The model under review builds one solid part; all positions refer to its coordinate system, in mm. A direction names the side the tool comes from. Coordinates: 2 decimals unless noted, no trailing zeros. Write each loop counter-clockwise with the first axis right and the second up, starting at its lowest first coordinate (ties: lowest second). Pieces come first, ordered by that corner, then holes.
1) Add section B-B, the plane y = -12.5. Give the number of separate pieces and of enclosed holes in the cut face, then the cut area to 3 significant figures.
2) For P1, Ø3, axis at y = -5, z = -3.5, coming from the -X side; P2, Ø4, axis at y = -12.5, z = -2, coming from the +X side; P3, Ø5.5, axis at x = 30.31, y = 17.5, coming from the -Z side, all flat-tipped, find the tip position at first contact; note any pin that passes through.
3) For line 1 (Y direction, x = -21.5, z = -2.5); line 2 (Y direction, x = 27, z = -5.5); line 3 (X direction, y = -12.5, z = -1.15), list the stretches that pass through material, from the lowest coordinate up.
4) Mouldability with a two-part tool opening along Y and no side actions: class faces 1 (the cylindrical face through (20.892, 15.917, -6.507)), 2 (the flat face through (0, 25, -3)), 3 (the cylindrical face through (-29.735, -24.471, -3.042)) as released by +Y, released by -Y, zero draft, split by the parting line, or undercut.
5) Add section A-A, the plane x = 0. State the section outline as (y, z) points, then the cut area to 3 significant figures.
6) Machinability: for faces 4 (the cylindrical face through (33.677, -2.103, -3.451)), 5 (the cylindrical face through (20.892, -9.083, -6.507)), which of the approach directions +Z, -Z, +X, -X, +Y, -Y give a long, thin tool a straight path to every point of the face, cutting with its end or side? Answer none if there is none.
from build123d import *

# Parameters (mm, degrees)
SKETCH020_R     = 10
SKETCH020_R_2   = 3.2
SKETCH020_R_3   = 1.7
SKETCH020_R_4   = 7
PAD_DEPTH       = 7
SKETCH021_R     = 3.5
POCKET_DEPTH    = 1
CHAMFER_SIZE    = 3.5
CHAMFER001_SIZE = 1.5
CHAMFER002_SIZE = 1.5
CHAMFER003_SIZE = 1.5
CHAMFER004_SIZE = 1.5
CHAMFER005_SIZE = 1.5
CHAMFER006_SIZE = 1.5
CHAMFER007_SIZE = 1.5
CHAMFER008_SIZE = 1.5
FILLET_R        = 5
FILLET001_R     = 5
FILLET002_R     = 5
FILLET003_R     = 5
FILLET004_R     = 1


with BuildPart() as part:
    # Sketch020 → Pad (new body)
    with BuildSketch(Plane(origin=(0, 0, 0), x_dir=(1, 0, 0), z_dir=(0, 0, -1))):
        with BuildLine():
            ThreePointArc((-29.933259, 25), (-39, 0), (-29.933259, -25))
            Line((-29.933259, -25), (29.933259, -25))
            ThreePointArc((29.933259, -25), (39, 0), (29.933259, 25))
            Line((-29.933259, 25), (29.933259, 25))
        make_face()
        Circle(SKETCH020_R, mode=Mode.SUBTRACT)
        with Locations((-32, 0)):
            Circle(SKETCH020_R_2, mode=Mode.SUBTRACT)
        with Locations((21.650635, 12.5)):
            Circle(SKETCH020_R_3, mode=Mode.SUBTRACT)
        with Locations((21.650635, -12.5)):
            Circle(SKETCH020_R_3, mode=Mode.SUBTRACT)
        with Locations((-21.650635, 12.5)):
            Circle(SKETCH020_R_3, mode=Mode.SUBTRACT)
        with Locations((-21.650635, -12.5)):
            Circle(SKETCH020_R_3, mode=Mode.SUBTRACT)
        with Locations((-30.310889, 17.5)):
            Circle(SKETCH020_R_3, mode=Mode.SUBTRACT)
        with Locations((-30.310889, -17.5)):
            Circle(SKETCH020_R_3, mode=Mode.SUBTRACT)
        with Locations((30.310889, 17.5)):
            Circle(SKETCH020_R_3, mode=Mode.SUBTRACT)
        with Locations((30.310889, -17.5)):
            Circle(SKETCH020_R_3, mode=Mode.SUBTRACT)
        with Locations((27, 0)):
            Circle(SKETCH020_R_4, mode=Mode.SUBTRACT)
    extrude(amount=PAD_DEPTH)

    # Sketch021 → Pocket (cut)
    with BuildSketch(Plane(origin=(0, 0, -7), x_dir=(1, 0, 0), z_dir=(0, 0, -1))):
        with Locations((21.650635, 12.5)):
            Circle(SKETCH021_R)
        with Locations((21.650635, -12.5)):
            Circle(SKETCH021_R)
        with Locations((-21.650635, 12.5)):
            Circle(SKETCH021_R)
        with Locations((-21.650635, -12.5)):
            Circle(SKETCH021_R)
    extrude(amount=-POCKET_DEPTH, mode=Mode.SUBTRACT)

    # Chamfer
    chamfer_edges = [part.edges().sort_by_distance(p)[0] for p in [
        (-35.2, 0, 0),
    ]]
    chamfer(chamfer_edges, length=CHAMFER_SIZE)

    # Chamfer001
    chamfer001_edges = [part.edges().sort_by_distance(p)[0] for p in [
        (-23.350635, -12.5, -6),
    ]]
    chamfer(chamfer001_edges, length=CHAMFER001_SIZE)

    # Chamfer002
    chamfer002_edges = [part.edges().sort_by_distance(p)[0] for p in [
        (-23.350635, 12.5, -6),
    ]]
    chamfer(chamfer002_edges, length=CHAMFER002_SIZE)

    # Chamfer003
    chamfer003_edges = [part.edges().sort_by_distance(p)[0] for p in [
        (19.950635, -12.5, -6),
    ]]
    chamfer(chamfer003_edges, length=CHAMFER003_SIZE)

    # Chamfer004
    chamfer004_edges = [part.edges().sort_by_distance(p)[0] for p in [
        (19.950635, 12.5, -6),
    ]]
    chamfer(chamfer004_edges, length=CHAMFER004_SIZE)

    # Chamfer005
    chamfer005_edges = [part.edges().sort_by_distance(p)[0] for p in [
        (-32.010889, 17.5, -7),
    ]]
    chamfer(chamfer005_edges, length=CHAMFER005_SIZE)

    # Chamfer006
    chamfer006_edges = [part.edges().sort_by_distance(p)[0] for p in [
        (-32.010889, -17.5, -7),
    ]]
    chamfer(chamfer006_edges, length=CHAMFER006_SIZE)

    # Chamfer007
    chamfer007_edges = [part.edges().sort_by_distance(p)[0] for p in [
        (28.610889, -17.5, -7),
    ]]
    chamfer(chamfer007_edges, length=CHAMFER007_SIZE)

    # Chamfer008
    chamfer008_edges = [part.edges().sort_by_distance(p)[0] for p in [
        (28.610889, 17.5, -7),
    ]]
    chamfer(chamfer008_edges, length=CHAMFER008_SIZE)

    # Fillet
    fillet_edges = [part.edges().sort_by_distance(p)[0] for p in [
        (-29.933259, 25, -3.5),
    ]]
    fillet(fillet_edges, radius=FILLET_R)

    # Fillet001
    fillet001_edges = [part.edges().sort_by_distance(p)[0] for p in [
        (29.933259, 25, -3.5),
    ]]
    fillet(fillet001_edges, radius=FILLET001_R)

    # Fillet002
    fillet002_edges = [part.edges().sort_by_distance(p)[0] for p in [
        (29.933259, -25, -3.5),
    ]]
    fillet(fillet002_edges, radius=FILLET002_R)

    # Fillet003
    fillet003_edges = [part.edges().sort_by_distance(p)[0] for p in [
        (-29.933259, -25, -3.5),
    ]]
    fillet(fillet003_edges, radius=FILLET003_R)

    # Fillet004
    fillet004_edges = [part.edges().sort_by_distance(p)[0] for p in [
        (0, 25, -7),
    ]]
    fillet(fillet004_edges, radius=FILLET004_R)


solid = part.part
Geometry results:
1. separate pieces: 3
1. enclosed holes: 0
1. area: 457 mm2
2. P1: stops at x = -38.84
2. P2: stops at x = 37.56
2. P3: stops at z = -6.55
3. line 1: y = -25 to -14.19, -10.81 to 10.81, 14.19 to 25
3. line 2: y = -25 to -7, 7 to 25
3. line 3: x = -36.94 to -23.35, -19.95 to 19.95, 23.35 to 36.94
4. face 1: undercut
4. face 2: released by +Y
4. face 3: released by -Y
5. outline: (-25, -6) arc R1 ccw to (-24, -7) - (-10, -7) - (-10, 0) - (-25, 0) - close; (10, -7) - (24, -7) arc R1 ccw to (25, -6) - (25, 0) - (10, 0) - close
5. area: 210 mm2
6. face 4: +Z, -Z
6. face 5: -Z
